Design review of the part built by this model. Coordinates are the model's own, in mm. A direction names the side the tool comes from. Round coordinates to 2 decimals unless told otherwise and drop trailing zeros. Loops run counter-clockwise (first coordinate to the right, second up) from the corner with the lowest first, then second, coordinate; pieces in that order, holes last. Notation, with made-up numbers: (8.5, 3.25) - (36.5, 3.25) arc R28 cw to (36.5, 33.25) - close; hole circle Ø3 at (12, 62). An arc over 180 degrees is marked (long way). Use one line per item in the form item = value. Start each with the question number.
(1) We need section A-A, the plane z = 71.5. Write out the cut boundary in (x, y), then the cut area to 3 significant figures.
(2) For pin 1 (1.5 mm diameter, centred on x = -0.5, z = 43.5, fed in from +Y); pin 2 (0.5 mm diameter, centred on y = 3, z = 71, fed in from +X); pin 3 (1.5 mm diameter, centred on x = 1, z = 38.5, fed in from +Y), all flat-tipped, find the tip position at first contact; note any pin that passes through.
(3) Wall thickness on probe 1 along Y at (x, z) = (0.15, 83); probe 2 along Y at (x, z) = (1.85, 22); probe 3 along X at (y, z) = (2.25, 18): over which ranges is each line inside the solid? List them lowest first. Write a range as [from, to].
(4) Machinability: for faces 1 (the flat face through (0.062, 1, 49)), 2 (the flat face through (0.963, 5.717, 49.3)), 3 (the flat face through (-1, 4, 0)), which of the approach directions +Z, -Z, +X, -X, +Y, -Y give a long, thin tool a straight path to every point of the face, cutting with its end or side? Answer none if there is none.
from build123d import *

# Parameters (mm, degrees)
EXTRUDE_1_DEPTH = 100


with BuildPart() as part:
    # 草图1 → 凸台-拉伸1 (new body)
    with BuildSketch(Plane.XY):
        with BuildLine():
            Line((1.910511393, 6.357959232), (-2.838177965, 7.757123338))
            Line((-2.838177965, 7.757123338), (-2.838177965, 7.373559769))
            Line((-2.838177965, 7.373559769), (-1.131654309, 3.630979973))
            Line((-1.131654309, 3.630979973), (-1.866356806, 3.881090486))
            Line((-1.866356806, 3.881090486), (-0.940400183, 2.396674584))
            Line((-0.940400183, 2.396674584), (-1.67510268, 2.646785097))
            Line((-1.67510268, 2.646785097), (-0.749146057, 1.162369196))
            Line((-0.749146057, 1.162369196), (-1.483848554, 1.412479708))
            Line((-1.483848554, 1.412479708), (-0.109115741, 0.02218372))
            ThreePointArc((-0.109115741, 0.02218372), (0, 0), (0.061991812, 0.092495284))
            Line((0.061991812, 0.092495284), (0.061991812, 1.893178292))
            Line((0.061991812, 1.893178292), (0.725818023, 2.227560058))
            Line((0.725818023, 2.227560058), (0.061991812, 2.561941824))
            Line((0.061991812, 2.561941824), (0.061991812, 3.512604418))
            Line((0.061991812, 3.512604418), (0.725818023, 3.846986184))
            Line((0.725818023, 3.846986184), (0.061991812, 4.18136795))
            Line((0.061991812, 4.18136795), (0.061991812, 5.461024264))
            Line((0.061991812, 5.461024264), (1.89024786, 5.980114276))
            ThreePointArc((1.89024786, 5.980114276), (2.035334753, 6.161799215), (1.910511393, 6.357959232))
        make_face()
    extrude(amount=EXTRUDE_1_DEPTH)


solid = part.part
Data:
q1.outline = (-2.84, 7.37) - (-1.13, 3.63) - (-1.87, 3.88) - (-0.94, 2.4) - (-1.68, 2.65) - (-0.75, 1.16) - (-1.48, 1.41) - (-0.11, 0.02) arc R0.1 ccw to (0.06, 0.09) - (0.06, 1.89) - (0.73, 2.23) - (0.06, 2.56) - (0.06, 3.51) - (0.73, 3.85) - (0.06, 4.18) - (0.06, 5.46) - (1.89, 5.98) arc R0.2 ccw to (1.91, 6.36) - (-2.84, 7.76) - close
q1.area = 13.9 mm^2
q2.pin_1 = 7.29
q2.pin_2 = 0.06
q2.pin_3 = 6.85
q3.probe_1 = [1.94, 2.52], [3.56, 4.14], [5.49, 6.88]
q3.probe_2 = [5.97, 6.38]
q3.probe_3 = [-1.43, 0.68]
q4.face_1 = +Z, -Z, +X, -Y
q4.face_2 = +Z, -Z, +X
q4.face_3 = -Z, +X, -X, +Y, -Y
